Autodesk Fusion 360 part; units mm, degrees
sketch "Sketch1" plane through (0, 0, 0) normal (0, 0, 1) x (1, 0, 0)
  line L0 (2.6252, 0) -> (7.4595, 0)
  line L1 (10.0424, 2.5828) -> (10.0424, 3.3)
  line L2 (0.0424, 3.3) -> (0.0424, 2.5828)
  line L3 (8.0424, 3.7) -> (8.0424, 4.8)
  line L4 (2.0424, 4.8) -> (2.0424, 3.7)
  line L5 (0.101, 2.4414) -> (2.4838, 0.0586)
  line L6 (0.0424, 2.5) -> (3.5052, 2.5) construction
  line L7 (5.0424, 3.5) -> (5.0424, 0) construction
  line L8 (9.9838, 2.4414) -> (7.601, 0.0586)
  line L9 (9.8424, 3.5) -> (8.2424, 3.5)
  line L10 (1.8424, 3.5) -> (0.2424, 3.5)
  line L11 (5.0424, 4.7) -> (5.3424, 5)
  line L12 (5.0424, 4.7) -> (6.213, 4.7) construction
  line L13 (5.0424, 4.7) -> (4.7424, 5)
  line L14 (5.0424, 4.7) -> (6.2088, 4.7) construction
  line L15 (7.8424, 5) -> (5.3424, 5)
  line L16 (4.7424, 5) -> (2.2424, 5)
  arc A0 (0.2424, 3.5) -> (0.0424, 3.3) centre (0.2424, 3.3) ccw
  arc A1 (0.0424, 2.5828) -> (0.101, 2.4414) centre (0.2424, 2.5828) ccw
  arc A2 (2.4838, 0.0586) -> (2.6252, 0) centre (2.6252, 0.2) ccw
  arc A3 (7.4595, 0) -> (7.601, 0.0586) centre (7.4595, 0.2) ccw
  arc A4 (9.9838, 2.4414) -> (10.0424, 2.5828) centre (9.8424, 2.5828) ccw
  arc A5 (10.0424, 3.3) -> (9.8424, 3.5) centre (9.8424, 3.3) ccw
  arc A6 (8.0424, 3.7) -> (8.2424, 3.5) centre (8.2424, 3.7) ccw
  arc A7 (8.0424, 4.8) -> (7.8424, 5) centre (7.8424, 4.8) ccw
  arc A8 (2.2424, 5) -> (2.0424, 4.8) centre (2.2424, 4.8) ccw
  arc A9 (1.8424, 3.5) -> (2.0424, 3.7) centre (1.8424, 3.7) ccw
  dimension "d1" = 10
  dimension "d4" = 5
  dimension "d5" = 45
  dimension "d6" = 1
  dimension "d7" = 5
  dimension "d8" = 6
  dimension "d9" = 2
  dimension "d10" = 2
  dimension "d12" = 45
  dimension "d13" = 0.3
  dimension "d14" = 5
  dimension "d15" = 1.5
  dimension "d16" = 0.2
extrude "Extrude1" add sketch "Sketch1" along normal blind 10
hole "Hole1" at (5.0424, 5, 5) direction (0, -1, 0) diameter 2.529 depth 5.834 tip angle 180 countersink diameter 4 countersink angle 90
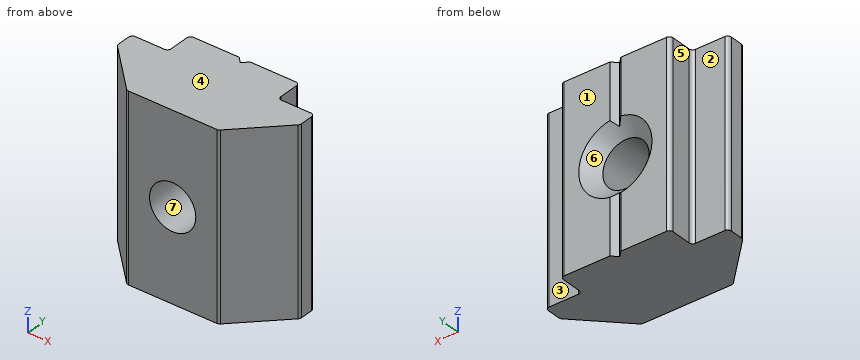
Here's how the part is built. I have some questions about the finished solid (model axes, mm). Face numbers are marked on the shaded views. A direction names the side the tool comes from. Coordinates: 2 decimals unless noted, no trailing zeros. Write each loop counter-clockwise with the first axis right and the second up, starting at its lowest first coordinate (ties: lowest second). Pieces come first, ordered by that corner, then holes.
Item 1: On a 3-axis mill with a long thin cutter (end or side, diameter ignored), from which of +Z, -Z, +X, -X, +Y, -Y can I reach the whole of each face in a straight line? I mean the marked faces 1, 2 and 3. Say none if no direction works.
Item 2: I want a section at A-A on z = 5. Write out the boundary of the cut face in (x, y), and give its area (3 significant figures).
Item 3: Will these pins go through, and if not, where does the flat tip stop? pin 1 (0.5 mm diameter, centred on x = 1, z = 3, fed in from +Y); pin 2 (0.5 mm diameter, centred on y = 4, z = 4.5, fed in from +X).
Item 4: If I drill on line 1 (X direction, y = 3.05, z = 5); line 2 (X direction, y = 1.15, z = 5); line 3 (Z direction, x = 5, y = 1.95), over which ranges is the centre line in solid material (lowest first)?
Item 5: I want a section at C-C on z = 2. Write out the boundary of the cut face in (x, y).
Item 6: I want a section at D-D on x = 9. Write out the boundary of the cut face in (y, z), and give its area (3 significant figures).
Item 7: I want a section at B-B on y = 3.15. Write out the boundary of the cut face in (x, z), and give its area (3 significant figures).
Item 8: If we mould it in two halves opening along Z, with no side actions, what happens to the marked faces 4, 5, 6 and 7? For each: +Z half, -Z half, draft (parallel to the pull), parting line (faces both ways), or undercut.
Findings below:
1. face 1: +Z, -Z, +X, -X, +Y
1. face 2: +Z, -Z, -X, +Y
1. face 3: +Z, -Z, +X, +Y
2. outline: (0.04, 2.58) arc R0.2 ccw to (0.1, 2.44) - (2.48, 0.06) arc R0.2 ccw to (2.63, 0) - (3.78, 0) - (3.78, 4.26) - (3.04, 5) - (2.24, 5) arc R0.2 ccw to (2.04, 4.8) - (2.04, 3.7) arc R0.2 cw to (1.84, 3.5) - (0.24, 3.5) arc R0.2 ccw to (0.04, 3.3) - close; (6.31, 0) - (7.46, 0) arc R0.2 ccw to (7.6, 0.06) - (9.98, 2.44) arc R0.2 ccw to (10.04, 2.58) - (10.04, 3.3) arc R0.2 ccw to (9.84, 3.5) - (8.24, 3.5) arc R0.2 cw to (8.04, 3.7) - (8.04, 4.8) arc R0.2 ccw to (7.84, 5) - (7.04, 5) - (6.31, 4.26) - close
2. area: 24.5 mm2
3. pin 1: stops at y = 3.5
3. pin 2: stops at x = 8.04
4. line 1: x = 0.04 to 3.78, 6.31 to 10.04
4. line 2: x = 1.39 to 3.78, 6.31 to 8.69
4. line 3: z = 0 to 3.74, 6.26 to 10
5. outline: (0.04, 2.58) arc R0.2 ccw to (0.1, 2.44) - (2.48, 0.06) arc R0.2 ccw to (2.63, 0) - (7.46, 0) arc R0.2 ccw to (7.6, 0.06) - (9.98, 2.44) arc R0.2 ccw to (10.04, 2.58) - (10.04, 3.3) arc R0.2 ccw to (9.84, 3.5) - (8.24, 3.5) arc R0.2 cw to (8.04, 3.7) - (8.04, 4.8) arc R0.2 ccw to (7.84, 5) - (5.34, 5) - (5.04, 4.7) - (4.74, 5) - (2.24, 5) arc R0.2 ccw to (2.04, 4.8) - (2.04, 3.7) arc R0.2 cw to (1.84, 3.5) - (0.24, 3.5) arc R0.2 ccw to (0.04, 3.3) - close
6. outline: (1.46, 0) - (3.5, 0) - (3.5, 10) - (1.46, 10) - close
6. area: 20.4 mm2
7. outline: (0.04, 0) - (10.04, 0) - (10.04, 10) - (0.04, 10) - close; hole circle Ø2.53 at (5.04, 5)
7. area: 95.0 mm2
8. face 4: +Z half
8. face 5: draft
8. face 6: undercut
8. face 7: undercut
